Here's how the part is built. I have some questions about the finished solid (model axes, mm). A direction names the side the tool comes from. Round coordinates to 2 decimals unless told otherwise and drop trailing zeros. Order: outer loops, then holes, each group sorted by start corner. A loop starts at its lowest first (then second) coordinate and runs counter-clockwise, first axis right, second up. Notation, with made-up numbers: (-1.5, 69) - (27.5, 69) arc R29 cw to (27.5, 99) - close; hole circle Ø2 at (46.25, 69.5). An arc over 180 degrees is marked (long way). Answer as a JSON object with one key per item and string values.
Autodesk Inventor part; units mm, degrees
ref_plane "YZ Plane" through (0, 0, 0) normal (1, 0, 0) x (0, 1, 0)
ref_plane "XZ Plane" through (0, 0, 0) normal (0, 1, 0) x (-1, 0, 0)
ref_plane "XY Plane" through (0, 0, 0) normal (0, 0, 1) x (1, 0, 0)
sketch "Sketch1" plane through (0, 0, 0) normal (0, 1, 0) x (-1, 0, 0)
  circle A0 centre (0, 0) radius 60
  dimension "d0" = 120
extrude "Extrusion1" add sketch "Sketch1" along normal blind 8
sketch "Sketch2" plane through (0, 8, 0) normal (0, 1, 0) x (1, 0, 0)
  circle A0 centre (-54, 0) radius 4
  circle A1 centre (-54, 0) radius 2.5
  circle A2 centre (0, -54) radius 4
  circle A3 centre (0, -54) radius 2.5
  circle A4 centre (54, 0) radius 4
  circle A5 centre (54, 0) radius 2.5
  circle A6 centre (0, 54) radius 4
  circle A7 centre (0, 54) radius 2.5
  point P0 (0, 0)
  dimension "d3" = 8
  dimension "d4" = 5
  dimension "d5" = 8
  dimension "d6" = 5
  dimension "d7" = 8
  dimension "d8" = 5
  dimension "d9" = 8
  dimension "d10" = 5
extrude "Extrusion2" cut sketch "Sketch2" against normal blind 8 contours A1 | A3 | A5 | A7
sketch "Sketch3" plane through (0, 8, 0) normal (0, 1, 0) x (1, 0, 0)
  circle A0 centre (-54, 0) radius 2.5
  circle A1 centre (-54, 0) radius 4
  circle A2 centre (-54, 0) radius 2.5
  circle A3 centre (0, 54) radius 2.5
  circle A4 centre (0, 54) radius 4
  circle A5 centre (0, 54) radius 2.5
  circle A6 centre (54, 0) radius 2.5
  circle A7 centre (54, 0) radius 4
  circle A8 centre (54, 0) radius 2.5
  circle A9 centre (0, -54) radius 4
  circle A10 centre (0, -54) radius 2.5
  point P0 (0, 0)
  dimension "d13" = 8
  dimension "d14" = 8
  dimension "d15" = 5
  dimension "d16" = 8
  dimension "d17" = 5
  dimension "d18" = 8
extrude "Extrusion3" cut sketch "Sketch3" against normal blind 3
sketch "Sketch4" plane through (0, 8, 0) normal (0, 1, 0) x (1, 0, 0)
  circle A0 centre (0, 0) radius 47.5
  circle A1 centre (0, 0) radius 45
  line L0 (0, 0) -> (-10, 0)
  line L1 (-10, 0) -> (-10, -9)
  line L2 (-10, -9) -> (0, -9)
  line L3 (0, -9) -> (0, 0)
  line L4 (0, -9) -> (10, -9)
  line L5 (10, -9) -> (10, 0)
  line L6 (10, 0) -> (0, 0)
  line L7 (0, 0) -> (0, -9)
  line L8 (-10, -9) -> (10, -9)
  line L9 (10, -9) -> (10, -16)
  line L10 (10, -16) -> (-10, -16)
  line L11 (-10, -16) -> (-10, -9)
  dimension "d21" = 95
  dimension "d22" = 90
  dimension "d23" = 10
  dimension "d24" = 9
  dimension "d25" = 10
  dimension "d26" = 7
extrude "Extrusion4" add sketch "Sketch4" along normal blind 47.5 contours A0
sketch "Sketch5" plane through (0, 8, 0) normal (0, 1, 0) x (1, 0, 0)
  line L0 (0, 0) -> (-10, 0)
  line L1 (-10, 0) -> (-10, -9)
  line L2 (-10, -9) -> (0, -9)
  line L3 (0, -9) -> (0, 0)
  line L4 (-10, -9) -> (10, -9)
  line L5 (10, -9) -> (10, -16)
  line L6 (10, -16) -> (-10, -16)
  line L7 (-10, -16) -> (-10, -9)
  line L8 (-10, -9) -> (10, -9)
  line L9 (10, -9) -> (10, 31)
  line L10 (10, 31) -> (-10, 31)
  line L11 (-10, 31) -> (-10, -9)
  line L12 (-10, 31) -> (-2, 31)
  line L13 (-2, 31) -> (-2, 38.36)
  line L14 (-2, 38.36) -> (-10, 38.36)
  line L15 (-10, 38.36) -> (-10, 31)
  line L16 (-10, 31) -> (10, 31)
  line L17 (10, 31) -> (10, 39)
  line L18 (10, 39) -> (-10, 39)
  line L19 (-10, 39) -> (-10, 31)
  line L20 (-10, -9) -> (10, -9)
  line L21 (10, -9) -> (10, -17)
  line L22 (10, -17) -> (-10, -17)
  line L23 (-10, -17) -> (-10, -9)
  dimension "d29" = 10
  dimension "d30" = 9
  dimension "d31" = 20
  dimension "d32" = 7
  dimension "d33" = 40
  dimension "d34" = 8
  dimension "d35" = 8
  dimension "d36" = 8
extrude "Extrusion5" add sketch "Sketch5" along normal blind 28 contours L4 L5 L6 L7 L2 | L15 L14 L13 L10 | L6 L21 L22 L23 | L13 L14 L19 L18 L17 L10
sketch "Sketch6" plane through (0, 36, 0) normal (0, 1, 0) x (1, 0, 0)
  line L0 (10, -17) -> (-10, -17)
  line L1 (-10, -9) -> (10, -9)
  line L2 (0, -17) -> (-4, -17)
  line L3 (-4, -17) -> (-4, -9)
  line L4 (-4, -9) -> (0, -9)
  line L5 (0, -9) -> (0, -17)
  line L6 (0, -17) -> (4, -17)
  line L7 (4, -17) -> (4, -9)
  line L8 (4, -9) -> (0, -9)
  line L9 (0, -9) -> (0, -17)
  point P0 (0, 0)
  dimension "d39" = 4
  dimension "d40" = 4
extrude "Extrusion6" cut sketch "Sketch6" against normal blind 28
sketch "Sketch7" plane through (0, 36, 0) normal (0, 1, 0) x (1, 0, 0)
  line L0 (-10, -17) -> (-4, -17)
  line L1 (4, -9) -> (10, -9)
  line L2 (-4, -17) -> (4, -17)
  line L3 (4, -17) -> (4, -9)
  line L4 (4, -9) -> (-4, -9)
  line L5 (-4, -9) -> (-4, -17)
  point P0 (0, 0)
extrude "Extrusion7" add sketch "Sketch7" against normal blind 22
sketch "Sketch8" plane through (0, 36, 0) normal (0, 1, 0) x (1, 0, 0)
  line L0 (-4, -17) -> (-10, -17)
  line L1 (10, -17) -> (10, -9)
  line L2 (-10, -17) -> (10, -17)
  line L3 (10, -17) -> (10, -15)
  line L4 (10, -15) -> (-10, -15)
  line L5 (-10, -15) -> (-10, -17)
  line L6 (-4, -9) -> (4, -9)
  line L7 (0, -9) -> (-5, -9)
  line L8 (-5, -9) -> (-5, -17)
  line L9 (-5, -17) -> (0, -17)
  line L10 (0, -17) -> (0, -9)
  line L11 (-10, -17) -> (10, -17)
  line L12 (0, -9) -> (5, -9)
  line L13 (5, -9) -> (5, -17)
  line L14 (5, -17) -> (0, -17)
  line L15 (0, -17) -> (0, -9)
  circle A0 centre (-5, -15) radius 2
  circle A1 centre (5, -15) radius 2
  line L16 (-10, 31) -> (-10, 39)
  line L17 (10, 39) -> (10, 31)
  line L18 (-10, 39) -> (10, 39)
  line L19 (10, 39) -> (10, 37)
  line L20 (10, 37) -> (-10, 37)
  line L21 (-10, 37) -> (-10, 39)
  line L22 (10, 31) -> (-10, 31)
  line L23 (-10, 39) -> (10, 39)
  line L24 (0, 31) -> (-5, 31)
  line L25 (-5, 31) -> (-5, 39)
  line L26 (-5, 39) -> (0, 39)
  line L27 (0, 39) -> (0, 31)
  line L28 (0, 31) -> (5, 31)
  line L29 (5, 31) -> (5, 39)
  line L30 (5, 39) -> (0, 39)
  line L31 (0, 39) -> (0, 31)
  circle A2 centre (-5, 37) radius 2
  circle A3 centre (5, 37) radius 2
  point P0 (0, 0)
  dimension "d45" = 2
  dimension "d46" = 5
  dimension "d47" = 5
  dimension "d48" = 4
  dimension "d49" = 4
  dimension "d50" = 2
  dimension "d51" = 4
  dimension "d52" = 4
extrude "Extrusion8" cut sketch "Sketch8" against normal blind 10 contours A0 L4 L8 | L8 L4 A0 | L8 A0 L4 | L4 A0 L8 | A1 L4 L13 | L13 L4 A1 | L13 A1 L4 | L4 A1 L13 | A2 L25 L20 | L20 L25 A2 | L25 L20 A2 | A2 L20 L25 | A3 L20 L29 | L29 L20 A3 | A3 L29 L20 | A3 L20 L29
properties part number "Base Part"
1. For P1, Ø1.5, axis at x = -10.5, y = 23.5, coming from the +Z side; P2, Ø2.5, axis at y = 22.5, z = -35, coming from the +X side; P3, Ø4, axis at y = 38, z = -21, coming from the +X side; P4, Ø4.5, axis at x = -54, z = 0, coming from the +Y side, each with a flat end and sliding along its axis, tell me the tip position at first contact or that it passes through.
Responses:
{"P1": "z = 46.49", "P2": "x = 33.42", "P3": "x = 43.53", "P4": "through"}
2. Imagine slicing it at A-A (y = 28.5). List the corners of the cut face in (x, z) for me, plus the area to 3 significant figures.
Responses:
{"outline": "circle Ø95 at (0, 0); (-10, -39) - (10, -39) - (10, -31) - (-10, -31) - close; (-10, 9) - (10, 9) - (10, 17) - (-10, 17) - close; hole circle Ø90 at (0, 0); hole circle Ø4 at (-5, -37); hole circle Ø4 at (-5, 15); hole circle Ø4 at (5, -37); hole circle Ø4 at (5, 15)", "area": "996 mm2"}
3. Imagine slicing it at D-D (z = 40). List the corners of the cut face in (x, y) for me.
Responses:
{"outline": "(-44.72, 0) - (44.72, 0) - (44.72, 8) - (25.62, 8) - (25.62, 55.5) - (20.62, 55.5) - (20.62, 8) - (-20.62, 8) - (-20.62, 55.5) - (-25.62, 55.5) - (-25.62, 8) - (-44.72, 8) - close"}
4. For faces 4 (the face through (57.815, 6.521, -1.201)), 5 (the face through (42, 55.5, 17)), 6 (the face through (-4, 11, 13)), which set-ups out of +Z, -Z, +X, -X, +Y, -Y let a thin tool reach every point of the face, with its end or its side?
Responses:
{"face 4": "+Y", "face 5": "+Z, -Z, +X, -X, +Y", "face 6": "none"}
5. Thinking about a two-plate mould opening in X: for faces 1 (the face through (-0.867, 6.521, 57.905)), 2 (the face through (-17, 8, 45)), 3 (the face through (-10.3, 31.42, -46.37)), which applies, pulls with the +X half, pulls with the -X half, needs draft (parallel to the pull), parting line crosses it, or undercut?
Responses:
{"face 1": "undercut", "face 2": "needs draft", "face 3": "parting line crosses it"}
6. Imagine slicing it at B-B (z = 0). List the corners of the cut face in (x, y) for me, plus the area to 3 significant figures.
Responses:
{"outline": "(-60, 0) - (-56.5, 0) - (-56.5, 5) - (-58, 5) - (-58, 8) - (-60, 8) - close; (-51.5, 0) - (51.5, 0) - (51.5, 5) - (50, 5) - (50, 8) - (47.5, 8) - (47.5, 55.5) - (45, 55.5) - (45, 8) - (-45, 8) - (-45, 55.5) - (-47.5, 55.5) - (-47.5, 8) - (-50, 8) - (-50, 5) - (-51.5, 5) - close; (56.5, 0) - (60, 0) - (60, 8) - (58, 8) - (58, 5) - (56.5, 5) - close", "area": "1,100 mm2"}
7. If I drill on L1, parallel to X at y = 20.5, z = -35; L2, parallel to X at y = 23.5, z = -32; L3, parallel to Y at x = -18.5, z = -19.5, over which ranges is the centre line in solid material (lowest first)? Write a range as [from, to].
Responses:
{"L1": "[-32.11, -28.28], [-10, 10], [28.28, 32.11]", "L2": "[-35.1, -31.64], [-10, 10], [31.64, 35.1]", "L3": "[0, 8]"}
8. Imagine slicing it at C-C (x = 54). List the corners of the cut face in (y, z) for me.
Responses:
{"outline": "(0, -26.15) - (8, -26.15) - (8, -4) - (5, -4) - (5, -2.5) - (0, -2.5) - close; (0, 2.5) - (5, 2.5) - (5, 4) - (8, 4) - (8, 26.15) - (0, 26.15) - close"}
